Geometry: final body of the model. Coordinates: model frame, mm. Face numbers are marked on the shaded views. A direction names the side the tool comes from. Give positions to 0.01 mm unless a question says otherwise; leave off trailing zeros. Write each loop counter-clockwise with the first axis right and the second up, starting at its lowest first coordinate (ties: lowest second). Pieces come first, ordered by that corner, then holes. Notation, with made-up numbers: M 57,10 L 75,10 A25 cw 75,29 Z; hole C 51,21 d4. An arc over 180 degrees is marked long. Use a Markdown table: item, result. Add a question column.
1) Draft query along Y for the marked faces 4, 5 and 6. Return one class per face: +Y half, -Y half, draft (parallel to the pull), parting line (faces both ways), or undercut.
2) Set-up query: the marked faces 1, 2 and 3. Return all of +Z, -Z, +X, -X, +Y, -Y with unobstructed straight access to the full face (end or side cutting, diameter ignored); none if empty.
3) Section A-A on x = 0. Return the cut outline in (y, z) (1 decimal), then the cut area to 3 significant figures.
4) Pin query (flat end, axial travel): pin 1 (3 mm diameter, centred on x = 5.5, y = -3.5, fed in from +Z); pin 2 (4 mm diameter, centred on x = 7, z = 4.5, fed in from -Y) (3 decimals); pin 3 (5.5 mm diameter, centred on y = -31.75, z = 10.91, fed in from +X); pin 4 (13 mm diameter, centred on x = 0, y = 1.5, fed in from -Z). Return the tip coordinate at first contact, or that it passes through.
5) Line query: line 1 (Y direction, x = 0, z = 19.5) (3 decimals); line 2 (X direction, y = 5, z = 18); line 3 (X direction, y = -28, z = 7.25) (3 decimals). Output: solid intervals per line, ascending.
6) Section D-D on z = 17. State how many separate pieces and enclosed holes the cut face has, then the cut area to 3 significant figures.
```python
from build123d import *

# Parameters (mm, degrees)
SKETCH1_W                      = 57.15
SKETCH1_H                      = 31.75
BOSS_EXTRUDE1_DEPTH            = 20.6375
SKETCH2_R                      = 11.1125
CUT_EXTRUDE1_DEPTH             = 6.985
SKETCH3_R                      = 8.255
CUT_EXTRUDE2_DEPTH             = 2.413
SKETCH4_R                      = 3.96875
CUT_EXTRUDE3_DEPTH             = 35.56692943
CUT_EXTRUDE4_START             = -4.7625
SKETCH6_R                      = 9.525
CUT_EXTRUDE4_DEPTH             = 30.80442943
SKETCH7_W                      = 9.525
SKETCH7_H                      = 20.6375
BOSS_EXTRUDE2_DEPTH            = 22.225
SKETCH9_R                      = 3.175
CUT_EXTRUDE5_DEPTH             = 72.719166938
FILLET1_R                      = 6.35
F_1_4_0_2500_DOWEL_HOLE1_D     = 6.35
F_1_4_0_2500_DOWEL_HOLE1_DEPTH = 9.525
F_1_4_0_2500_DOWEL_HOLE1_TIP   = 1.907732465
FILLET3_R                      = 6.35
CHAMFER1_SIZE                  = 19.05


with BuildPart() as part:
    # Sketch1 → Boss-Extrude1 (new body)
    with BuildSketch(Plane.XY):
        Rectangle(SKETCH1_W, SKETCH1_H)
    extrude(amount=BOSS_EXTRUDE1_DEPTH)

    # Sketch2 → Cut-Extrude1 (cut)
    with BuildSketch(Plane(origin=(0, 0, 0), x_dir=(-1, 0, 0), z_dir=(0, 0, -1))):
        Circle(SKETCH2_R)
    extrude(amount=-CUT_EXTRUDE1_DEPTH, mode=Mode.SUBTRACT)

    # Sketch3 → Cut-Extrude2 (cut)
    with BuildSketch(Plane(origin=(0, 0, 6.985), x_dir=(-1, 0, 0), z_dir=(0, 0, -1))):
        Circle(SKETCH3_R)
    extrude(amount=-CUT_EXTRUDE2_DEPTH, mode=Mode.SUBTRACT)

    # Sketch4 → Cut-Extrude3 (cut, through all)
    with BuildSketch(Plane(origin=(0, 0, 9.398), x_dir=(-1, 0, 0), z_dir=(0, 0, -1))):
        Circle(SKETCH4_R)
    extrude(amount=-CUT_EXTRUDE3_DEPTH, mode=Mode.SUBTRACT)

    # Sketch6 → Cut-Extrude4 (cut, through all)
    with BuildSketch(Plane(origin=(0, 0, 9.398), x_dir=(-1, 0, 0), z_dir=(0, 0, -1)).offset(CUT_EXTRUDE4_START)):
        Circle(SKETCH6_R)
    extrude(amount=-CUT_EXTRUDE4_DEPTH, mode=Mode.SUBTRACT)

    # Sketch7 → Boss-Extrude2 (add)
    with BuildSketch(Plane.XZ.offset(15.875)):
        with Locations((-23.8125, 10.31875)):
            Rectangle(SKETCH7_W, SKETCH7_H)
        with Locations((23.8125, 10.31875)):
            Rectangle(SKETCH7_W, SKETCH7_H)
    extrude(amount=BOSS_EXTRUDE2_DEPTH)

    # Sketch9 → Cut-Extrude5 (cut, through all)
    with BuildSketch(Plane(origin=(28.575, 0, 0), x_dir=(0, 0, -1), z_dir=(1, 0, 0))):
        with Locations((-10.909520599, -31.75)):
            Circle(SKETCH9_R)
    extrude(amount=-CUT_EXTRUDE5_DEPTH, mode=Mode.SUBTRACT)

    # Fillet1
    fillet1_edges = [part.edges().sort_by_distance(p)[0] for p in [
        (-19.05, -15.875, 10.31875),
        (19.05, -15.875, 10.31875),
    ]]
    fillet(fillet1_edges, radius=FILLET1_R)

    # 1/4 (0.2500) Dowel Hole1
    with Locations(Plane.XY.offset(20.6375)):
        with Locations((-14.287572867, -0.8255), (14.287427022, -0.828020391)):
            Hole(F_1_4_0_2500_DOWEL_HOLE1_D / 2, depth=F_1_4_0_2500_DOWEL_HOLE1_DEPTH)
            with Locations((0, 0, -(F_1_4_0_2500_DOWEL_HOLE1_DEPTH + F_1_4_0_2500_DOWEL_HOLE1_TIP / 2))):  # 118° drill point
                Cone(0, F_1_4_0_2500_DOWEL_HOLE1_D / 2, F_1_4_0_2500_DOWEL_HOLE1_TIP, mode=Mode.SUBTRACT)

    # Fillet3
    fillet3_edges = [part.edges().sort_by_distance(p)[0] for p in [
        (-23.8125, -38.1, 0),
        (-23.8125, -38.1, 20.6375),
        (23.8125, -38.1, 20.6375),
        (23.8125, -38.1, 0),
    ]]
    fillet(fillet3_edges, radius=FILLET3_R)

    # Chamfer1
    chamfer1_edges = [part.edges().sort_by_distance(p)[0] for p in [
        (-28.575, 15.875, 10.31875),
        (28.575, 15.875, 10.31875),
    ]]
    chamfer(chamfer1_edges, length=CHAMFER1_SIZE)


solid = part.part
```
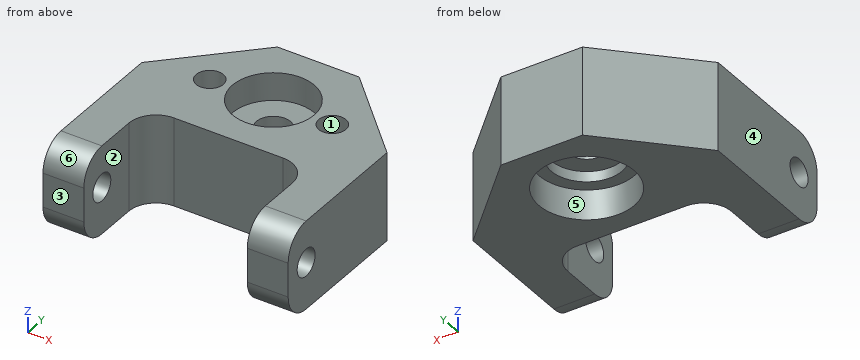
Found:
| question | item | result |
|---|---|---|
| 1 | face 4 | draft |
| 1 | face 5 | undercut |
| 1 | face 6 | -Y half |
| 2 | face 1 | +Z |
| 2 | face 2 | +Z, -Z, -Y |
| 2 | face 3 | +Z, -Z, +X, -X, -Y |
| 3 | outline | M -15.9,0 L -11.1,0 L -11.1,7 L -8.3,7 L -8.3,9.4 L -4,9.4 L -4,14.2 L -9.5,14.2 L -9.5,20.6 L -15.9,20.6 Z; M 4,9.4 L 8.3,9.4 L 8.3,7 L 11.1,7 L 11.1,0 L 15.9,0 L 15.9,20.6 L 9.5,20.6 L 9.5,14.2 L 4,14.2 Z |
| 3 | area | 299 mm² |
| 4 | pin 1 | z = 14.16 |
| 4 | pin 2 | y = -15.875 |
| 4 | pin 3 | through |
| 4 | pin 4 | z = 9.4 |
| 5 | line 1 | -15.875 to -9.525, 9.525 to 15.875 |
| 5 | line 2 | -20.4 to -8.11, 8.11 to 20.4 |
| 5 | line 3 | -28.575 to -19.05, 19.05 to 28.575 |
| 6 | separate pieces | 1 |
| 6 | enclosed holes | 3 |
| 6 | area | 1,530 mm² |
